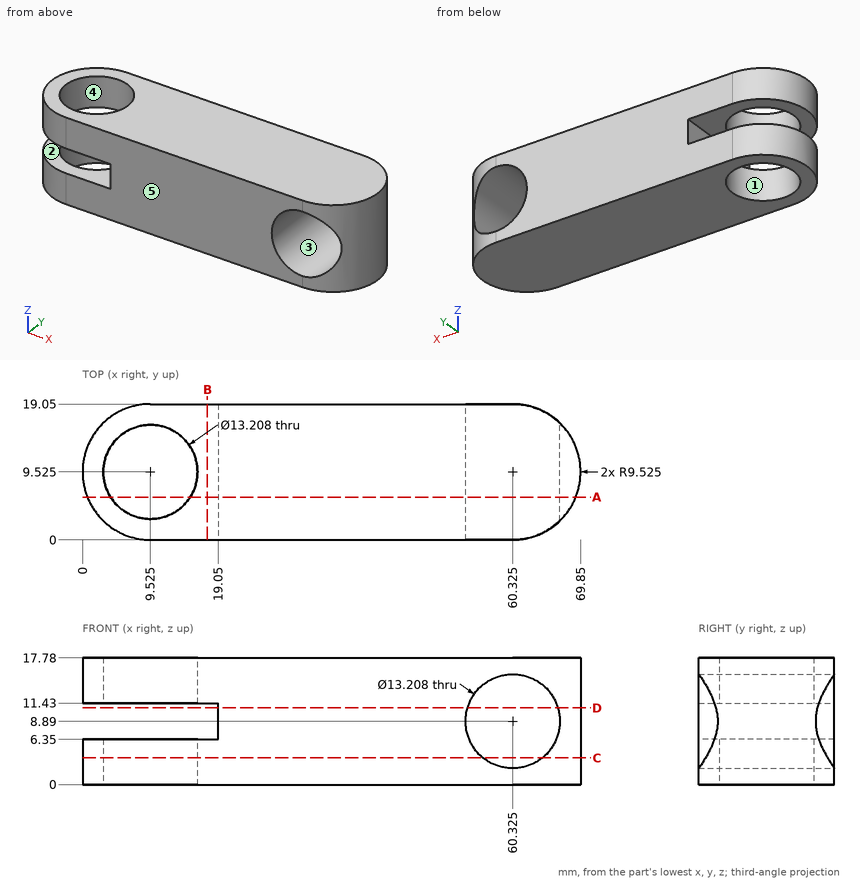
Design review of the part shown in the three views and the two pictorial views. Dimensions are in mm from the part's minimum x, y and z. A direction names the side the tool comes from. Round coordinates to 2 decimals unless told otherwise and drop trailing zeros. Write each loop counter-clockwise with the first axis right and the second up, starting at its lowest first coordinate (ties: lowest second). Pieces come first, ordered by that corner, then holes. Notation, with made-up numbers: (-20, 67) - (21, 67) arc R21 cw to (21, 94) - close; hole circle Ø8 at (-15.5, 48.25). An arc over 180 degrees is marked (long way). Return JSON: item names as keys, results as strings. Group by question number.
Item 1: We need section B-B on x = 17.5. Write out the cut boundary in (y, z).
Item 2: The part is to be moulded in two halves that separate along Y. For the marked faces 3, 4 and 5, say which applies: pulls with the +Y half, pulls with the -Y half, needs draft (parallel to the pull), parting line crosses it, or undercut.
Item 3: We need section A-A on y = 6. Write out the cut boundary in (x, z) (3 decimals), and give its area (3 significant figures).
Item 4: Insertion check: P1, Ø2, axis at y = 8, z = 3.5, coming from the +X side; P2, Ø2, axis at y = 17, z = 5, coming from the +X side; P3, Ø1.5, axis at y = 12, z = 8.5, coming from the -X side. Each pin has a flat end and moves straight along its axis. Give the tip position at first contact, or say it passes through.
Item 5: We need section D-D on z = 10.75. Write out the cut boundary in (x, y) (3 decimals), and give its area (3 significant figures).
Item 6: We need section C-C on z = 3.75. Write out the cut boundary in (x, y) (3 decimals), and give its area (3 significant figures).
Item 7: For probe 1 along Z at (x, y) = (60, 11.5); probe 2 along X at (y, z) = (15.25, 14); probe 3 along Z at (x, y) = (18.5, 16.25), list the stretches that pass through material, from the lowest coordinate up. Write a range as [from, to].
Item 8: Machinability: for the marked faces 1 and 2, which of the approach directions +Z, -Z, +X, -X, +Y, -Y give a long, thin tool a straight path to every point of the face, cutting with its end or side? Answer none if there is none.
Model answer:
{
 "1": {"outline": "(0, 0) - (19.05, 0) - (19.05, 6.35) - (0, 6.35) - close; (0, 11.43) - (19.05, 11.43) - (19.05, 17.78) - (0, 17.78) - close"},
 "2": {"face 3": "needs draft", "face 4": "undercut", "face 5": "pulls with the -Y half"},
 "3": {"outline": "(0.676, 0) - (3.94, 0) - (3.94, 6.35) - (0.676, 6.35) - close; (0.676, 11.43) - (3.94, 11.43) - (3.94, 17.78) - (0.676, 17.78) - close; (15.11, 0) - (69.174, 0) - (69.174, 17.78) - (15.11, 17.78) - (15.11, 11.43) - (19.05, 11.43) - (19.05, 6.35) - (15.11, 6.35) - close; hole circle Ø13.208 at (60.325, 8.89)", "area": "846 mm²"},
 "4": {"P1": "stops at x = 69.84", "P2": "stops at x = 67.31", "P3": "stops at x = 19.05"},
 "5": {"outline": "(19.05, 0) - (53.988, 0) - (53.988, 19.05) - (19.05, 19.05) - close; (66.662, 2.414) arc R9.525 ccw to (66.662, 16.636) - close", "area": "697 mm²"},
 "6": {"outline": "(9.525, 0) - (56.179, 0) - (56.179, 19.05) - (9.525, 19.05) arc R9.525 ccw to start; (64.471, 0.95) arc R9.525 ccw to (64.471, 18.1) - close; hole circle Ø13.208 at (9.525, 9.525)", "area": "960 mm²"},
 "7": {"probe 1": "z = [0, 2.29], [15.49, 17.78]", "probe 2": "x = [1.91, 6.23], [12.82, 56.14], [64.51, 67.94]", "probe 3": "z = [0, 6.35], [11.43, 17.78]"},
 "8": {"face 1": "+Z, -Z", "face 2": "-X, +Y, -Y"}
}
